For this review, take the finished solid that the model builds, in its own axes (mm). A direction names the side the tool comes from. Coordinates: 2 decimals unless noted, no trailing zeros. Write each loop counter-clockwise with the first axis right and the second up, starting at its lowest first coordinate (ties: lowest second). Pieces come first, ordered by that corner, then holes. Notation, with made-up numbers: (39.5, -1) - (68.5, -1) arc R27 ccw to (68.5, 24) - close; hole circle Ø3 at (37.5, -13). An arc over 180 degrees is marked (long way). Use one line per item in the form item = value. Start each with the question number.
1) We need section B-B (z = -1.05). Count the separate pieces of the cut face and the enclosed holes in it, plus the area to 3 significant figures.
2) For L1, parallel to Y at x = 0, z = -0.9; L2, parallel to X at y = -24.5, z = -0.95; L3, parallel to X at y = 265, z = 0.15, list the stretches that pass through material, from the lowest coordinate up. Write a range as from..to.
3) Mouldability with a two-part tool opening along Y and no side actions: class faces 3 (the cylindrical face through (-228.606, 304.241, 0.022)), 4 (the cylindrical face through (228.606, 305.359, 0.022)), 5 (the flat face through (9, -5, 1.588)) as pulls with the +Y half, pulls with the -Y half, needs draft (parallel to the pull), parting line crosses it, or undercut.
4) We need section A-A (x = -273). Give the boundary of the cut face in (y, z), plus the area to 3 significant figures.
5) Insertion check: P1, Ø5.5, axis at x = 215.9, y = -190.5, coming from the -Z side. The pin has a flat end and moves straight along its axis. Give the tip position at first contact, or say it passes through.
6) Tool access review of faces 1 (the flat face through (9, -5, -1.588)), 2 (the cylindrical face through (-406.394, 305.359, 0.022)): name each direction out of +Z, -Z, +X, -X, +Y, -Y from which nothing blocks a thin tool from reaching the whole face with its end or side.
```python
from build123d import *

# Parameters (mm, degrees)
F0_W     = 762
F0_H     = 3.175
F1_DEPTH = 647.7
F3_D     = 11.1125
F5_DEPTH = 3.175
F7_D     = 9.525


with BuildPart() as f1:
    # F0 (on Right) → F1 (new body, symmetric)
    with BuildSketch(Plane.YZ):
        Rectangle(F0_W, F0_H)
    extrude(amount=F1_DEPTH, both=True)

    # F3 (through all)
    with Locations(Plane.XY.offset(1.5875)):
        with Locations((463.55, 228.6), (463.55, 190.5), (463.55, -177.8), (463.55, -215.9), (0, 228.6), (0, 190.5), (0, -177.8), (0, -215.9), (-463.55, 190.5), (-463.55, 228.6), (-463.55, -177.8), (-463.55, -215.9)):
            Hole(F3_D / 2)

    # F4 (on face) → F5 (cut, through all)
    with BuildSketch(Plane.XY.offset(1.5875)):
        with BuildLine():
            ThreePointArc((254, 330.2), (228.6, 304.8), (254, 279.4))
            Line((254, 279.4), (381, 279.4))
            ThreePointArc((381, 279.4), (406.4, 304.8), (381, 330.2))
            Line((381, 330.2), (254, 330.2))
        make_face()
        with BuildLine():
            ThreePointArc((-381, 330.2), (-406.4, 304.8), (-381, 279.4))
            Line((-381, 279.4), (-254, 279.4))
            ThreePointArc((-254, 279.4), (-228.6, 304.8), (-254, 330.2))
            Line((-254, 330.2), (-381, 330.2))
        make_face()
    extrude(amount=-F5_DEPTH, mode=Mode.SUBTRACT)

    # F7 (through all)
    with Locations(Plane.XY.offset(1.5875)):
        with Locations((571.5, 304.8), (571.5, 263.525), (571.5, 222.25), (571.5, 180.975), (571.5, 139.7), (571.5, 98.425), (571.5, 15.875), (571.5, -149.225), (571.5, -273.05), (571.5, -231.775), (571.5, -190.5), (571.5, -66.675), (571.5, -107.95), (571.5, -25.4), (571.5, 57.15), (215.9, 98.425), (215.9, 139.7), (215.9, 180.975), (215.9, 222.25), (215.9, 263.525), (215.9, 57.15), (215.9, -25.4), (215.9, 15.875), (215.9, -107.95), (215.9, -66.675), (215.9, -149.225), (215.9, -190.5), (215.9, -231.775), (215.9, -273.05), (215.9, 304.8)):
            Hole(F7_D / 2)


solid = f1.part
```
Determined:
q1.separate_pieces = 1
q1.enclosed_holes = 44
q1.area = 967,000 mm²
q2.L1 = -381..-221.46, -210.34..-183.36, -172.24..184.94, 196.06..223.04, 234.16..381
q2.L2 = -647.7..211.22, 220.58..566.82, 576.18..647.7
q2.L3 = -647.7..211.37, 220.43..566.97, 576.03..647.7
q3.face_3 = undercut
q3.face_4 = undercut
q3.face_5 = needs draft
q4.outline = (-381, -1.59) - (279.4, -1.59) - (279.4, 1.59) - (-381, 1.59) - close; (330.2, -1.59) - (381, -1.59) - (381, 1.59) - (330.2, 1.59) - close
q4.area = 2,260 mm²
q5.P1 = through
q6.face_1 = -Z, +X, -X, +Y, -Y
q6.face_2 = +Z, -Z
